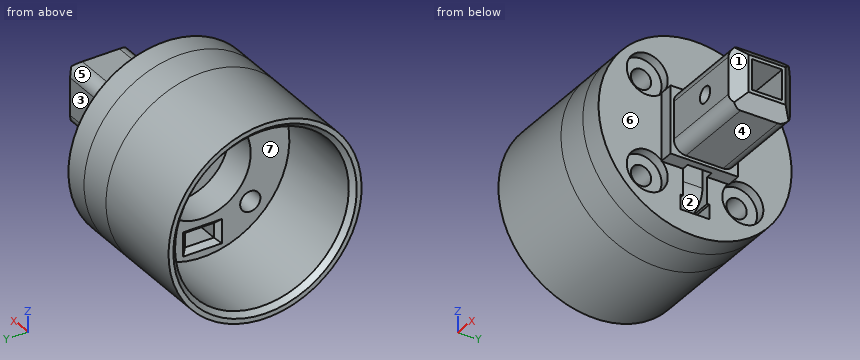
from build123d import *

# Parameters (mm, degrees)
SKETCH_1_R               = 20
EXTRUDE_1_DEPTH          = 5
SKETCH_2_W               = 6.3
SKETCH_2_H               = 6.3
CUT_EXTRUDE_1_DEPTH      = 5
EXTRUDE_START            = 7
SKETCH_4_R               = 20
SKETCH_4_R_2             = 10
EXTRUDE_2_DEPTH          = 7
CUT_EXTRUDE_2_DEPTH      = 20
CUT_EXTRUDE_2_DEPTH_BACK = 20
SKETCH_3_R               = 2.1
SKETCH_5_W               = 3
SKETCH_5_H               = 6
CUT_EXTRUDE_3_DEPTH      = 13
CHAMFER_1_SIZE           = 1
EXTRUDE_START_2          = 20
SKETCH_6_R               = 20
SKETCH_6_R_2             = 18
EXTRUDE_3_DEPTH          = 20
CHAMFER_2_SIZE           = 1
SKETCH_7_R               = 4.25
CUT_EXTRUDE_4_DEPTH      = 2
SKETCH_8_W               = 14
SKETCH_8_H               = 14
EXTRUDE_4_DEPTH          = 3
SKETCH_9_W               = 6.3
SKETCH_9_H               = 6.3
CUT_EXTRUDE_5_DEPTH      = 10
CUT_EXTRUDE_6_DEPTH      = 6
CUT_EXTRUDE_6_DEPTH_BACK = 5
SKETCH_10_W              = 3
SKETCH_10_H              = 5
FILLET_1_R               = 4
FILLET_2_R               = 2
SKETCH_11_W              = 12.7
SKETCH_11_H              = 12.7
SKETCH_11_W_2            = 6.3
SKETCH_11_H_2            = 6.3
EXTRUDE_5_DEPTH          = 20
CHAMFER_3_SIZE           = 2.5
SKETCH_12_R              = 1.65
CUT_EXTRUDE_7_DEPTH      = 20
FILLET_3_R               = 2.5


with BuildPart() as part:
    # 草图1 → 凸台-拉伸1 (new body)
    with BuildSketch(Plane(origin=(0, 0, 0), x_dir=(0, 0, -1), z_dir=(1, 0, 0))):
        Circle(SKETCH_1_R)
    extrude(amount=EXTRUDE_1_DEPTH)

    # 草图2 → 切除-拉伸1 (cut)
    with BuildSketch(Plane(origin=(5, 0, 0), x_dir=(0, 0, -1), z_dir=(1, 0, 0))):
        Rectangle(SKETCH_2_W, SKETCH_2_H)
    extrude(amount=-CUT_EXTRUDE_1_DEPTH, mode=Mode.SUBTRACT)

    # 草图4 → 凸台-拉伸2 (add)
    with BuildSketch(Plane.ZY.offset(EXTRUDE_START)):
        Circle(SKETCH_4_R)
        Circle(SKETCH_4_R_2, mode=Mode.SUBTRACT)
    extrude(amount=-EXTRUDE_2_DEPTH)

    # 草图3 → 切除-拉伸2 (cut, two sides: drawn at the far end of the back side and taken through both)
    with BuildSketch(Plane.ZY.offset(-CUT_EXTRUDE_2_DEPTH_BACK)):
        with Locations(Location((9.899494937, -9.899494937, 0), (0, 0, 180))):
            Circle(SKETCH_3_R)
        with Locations(Location((-9.899494937, -9.899494937, 0), (0, 0, 180))):
            Circle(SKETCH_3_R)
        with Locations(Location((-9.899494937, 9.899494937, 0), (0, 0, 180))):
            Circle(SKETCH_3_R)
        with Locations(Location((9.899494937, 9.899494937, 0), (0, 0, 180))):
            Circle(SKETCH_3_R)
    extrude(amount=CUT_EXTRUDE_2_DEPTH + CUT_EXTRUDE_2_DEPTH_BACK, mode=Mode.SUBTRACT)

    # 草图5 → 切除-拉伸3 (cut)
    with BuildSketch(Plane(origin=(5, 0, 0), x_dir=(0, 0, -1), z_dir=(1, 0, 0))):
        with Locations((14, 0)):
            Rectangle(SKETCH_5_W, SKETCH_5_H)
    extrude(amount=-CUT_EXTRUDE_3_DEPTH, mode=Mode.SUBTRACT)

    # 倒角1
    chamfer_1_edges = [part.edges().sort_by_distance(p)[0] for p in [
        (-7, -3, -14),
        (-7, 0, -15.5),
        (-7, 3, -14),
        (-7, 0, -12.5),
    ]]
    chamfer(chamfer_1_edges, length=CHAMFER_1_SIZE)

    # 草图6 → 凸台-拉伸3 (add)
    with BuildSketch(Plane.ZY.offset(7).offset(EXTRUDE_START_2)):
        Circle(SKETCH_6_R)
        Circle(SKETCH_6_R_2, mode=Mode.SUBTRACT)
    extrude(amount=-EXTRUDE_3_DEPTH)

    # 倒角2
    chamfer_2_edges = [part.edges().sort_by_distance(p)[0] for p in [
        (-27, 0, -18),
    ]]
    chamfer(chamfer_2_edges, length=CHAMFER_2_SIZE)

    # 草图7 → 切除-拉伸4 (cut)
    with BuildSketch(Plane(origin=(5, 0, 0), x_dir=(0, 0, -1), z_dir=(1, 0, 0))):
        with Locations((-9.899494937, 9.899494937)):
            Circle(SKETCH_7_R)
        with Locations((9.899494937, 9.899494937)):
            Circle(SKETCH_7_R)
        with Locations((9.899494937, -9.899494937)):
            Circle(SKETCH_7_R)
        with Locations((-9.899494937, -9.899494937)):
            Circle(SKETCH_7_R)
    extrude(amount=-CUT_EXTRUDE_4_DEPTH, mode=Mode.SUBTRACT)

    # 草图8 → 凸台-拉伸4 (add)
    with BuildSketch(Plane(origin=(5, 0, 0), x_dir=(0, 0, -1), z_dir=(1, 0, 0))):
        Rectangle(SKETCH_8_W, SKETCH_8_H)
    extrude(amount=EXTRUDE_4_DEPTH)

    # 草图9 → 切除-拉伸5 (cut)
    with BuildSketch(Plane.ZY.offset(-5)):
        Rectangle(SKETCH_9_W, SKETCH_9_H)
    extrude(amount=-CUT_EXTRUDE_5_DEPTH, mode=Mode.SUBTRACT)

    # 草图10 → 切除-拉伸6 (cut, two sides: drawn at the far end of the back side and taken through both)
    with BuildSketch(Plane(origin=(0, 0, -7), x_dir=(-1, 0, 0), z_dir=(0, 0, -1)).offset(-CUT_EXTRUDE_6_DEPTH_BACK)):
        with Locations((-5, 0)):
            Rectangle(SKETCH_10_W, SKETCH_10_H)
    extrude(amount=CUT_EXTRUDE_6_DEPTH + CUT_EXTRUDE_6_DEPTH_BACK, mode=Mode.SUBTRACT)

    # 圆角1
    fillet_1_edges = [part.edges().sort_by_distance(p)[0] for p in [
        (3.5, 0, -12.5),
    ]]
    fillet(fillet_1_edges, radius=FILLET_1_R)

    # 圆角2
    # the kernel refuses this fillet: 2 mm, written as the material it takes off along each edge
    with BuildSketch(Plane(origin=(6.5, 2.5, -3.15), x_dir=(1, 0, 0), z_dir=(0, -1, 0))) as fillet_2_piece_1:
        with BuildLine():
            CenterArc((FILLET_2_R, -FILLET_2_R), FILLET_2_R, 90, 90)
            Line((0, -FILLET_2_R), (0, 0))
            Line((0, 0), (FILLET_2_R, 0))
        make_face()
    extrude(amount=5, mode=Mode.SUBTRACT)

    # 草图11 → 凸台-拉伸5 (add)
    with BuildSketch(Plane(origin=(8, 0, 0), x_dir=(0, 0, -1), z_dir=(1, 0, 0))):
        Rectangle(SKETCH_11_W, SKETCH_11_H)
        Rectangle(SKETCH_11_W_2, SKETCH_11_H_2, mode=Mode.SUBTRACT)
    extrude(amount=EXTRUDE_5_DEPTH)

    # 倒角3
    chamfer_3_edges = [part.edges().sort_by_distance(p)[0] for p in [
        (28, 0, 6.35),
        (28, -6.35, 0),
        (28, 0, -6.35),
        (28, 6.35, 0),
    ]]
    chamfer(chamfer_3_edges, length=CHAMFER_3_SIZE)

    # 草图12 → 切除-拉伸7 (cut)
    with BuildSketch(Plane.XZ.offset(6.35)):
        with Locations(Location((18, 0, 0), (0, 0, 270))):
            Circle(SKETCH_12_R)
    extrude(amount=-CUT_EXTRUDE_7_DEPTH, mode=Mode.SUBTRACT)

    # 圆角3
    fillet_3_edges = [part.edges().sort_by_distance(p)[0] for p in [
        (16.75, 6.35, 6.35),
        (16.75, 6.35, -6.35),
        (16.75, -6.35, -6.35),
        (16.75, -6.35, 6.35),
    ]]
    fillet(fillet_3_edges, radius=FILLET_3_R)


solid = part.part
The listing builds one solid part. Answer for the finished solid, in the listing's coordinates (mm). Face numbers are marked on the shaded views. A direction names the side the tool comes from. Coordinates: 2 decimals unless noted, no trailing zeros. Order: outer loops, then holes, each group sorted by start corner. A loop starts at its lowest first (then second) coordinate and runs counter-clockwise, first axis right, second up.
Q1. A cutting plane is placed at D-D, the plane x = -13. Write down the section's boundary in (y, z).
Q2. Which of the six approach directions +Z, -Z, +X, -X, +Y, -Y give full straight-line access (tool end or side, diameter ignored) to the marked faces 4, 5, 6 and 7?
Q3. A cutting plane is placed at B-B, the plane y = 0. State how many separate pieces and enclosed holes the cut face has, and give its area (3 significant figures).
Q4. Consider line 1 (Y direction, x = -12.5, z = 0); line 2 (X direction, y = -2.5, z = 8); line 3 (X direction, y = 17, z = 3). Determine where each line is inside the solid, lowest interval first.
Q5. A cutting plane is placed at A-A, the plane x = 18. Write down the section's boundary in (y, z).
Q6. Given P1, Ø8, axis at x = 5.5, y = -14, coming from the -Z side; P2, Ø6, axis at x = 6.5, y = -2.5, coming from the +Z side; P3, Ø4, axis at x = 13, z = -1.5, coming from the -Y side; P4, Ø8, axis at x = -4, z = -0.5, coming from the +Y side, each flat-ended and moving along its own axis, determine where each tip first touches the part or whether it passes through.
Q7. For a pull along Y with two mould halves and no side action, classify the marked faces 1, 2 and 3 as pulls with the +Y half, pulls with the -Y half, needs draft (parallel to the pull), parting line crosses it, or undercut.
Answers follow:
1. outline: circle Ø40 at (0, 0); hole circle Ø36 at (0, 0)
2. face 4: -Z, +X, +Y, -Y
2. face 5: +Z, +X, +Y
2. face 6: +X
2. face 7: -X
3. separate pieces: 4
3. enclosed holes: 0
3. area: 471 mm2
4. line 1: y = -20 to -18, 18 to 20
4. line 2: x = 0 to 5
4. line 3: x = -7 to 5
5. outline: (-6.35, -3.85) arc R2.5 ccw to (-3.85, -6.35) - (3.85, -6.35) arc R2.5 ccw to (6.35, -3.85) - (6.35, -1.65) - (3.15, -1.65) - (3.15, -3.15) - (-3.15, -3.15) - (-3.15, -1.65) - (-6.35, -1.65) - close; (-6.35, 1.65) - (-3.15, 1.65) - (-3.15, 3.15) - (3.15, 3.15) - (3.15, 1.65) - (6.35, 1.65) - (6.35, 3.85) arc R2.5 ccw to (3.85, 6.35) - (-3.85, 6.35) arc R2.5 ccw to (-6.35, 3.85) - close
6. P1: stops at z = -17.3
6. P2: stops at z = 20
6. P3: stops at y = -6.35
6. P4: stops at y = 20
7. face 1: pulls with the -Y half
7. face 2: undercut
7. face 3: pulls with the +Y half
